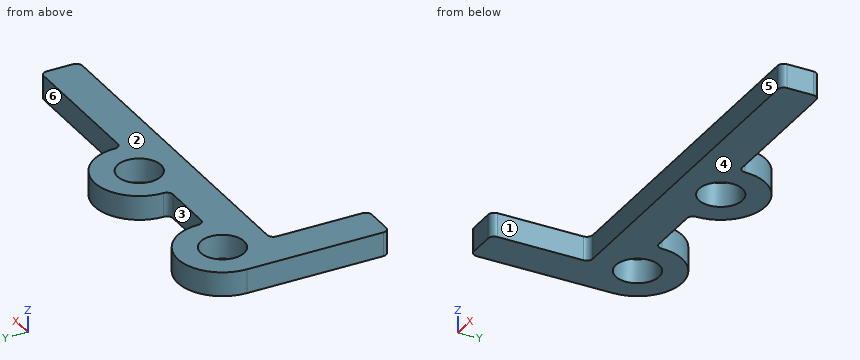
from build123d import *

# Parameters (mm, degrees)
SKETCH005_R = 1.8
PAD_DEPTH   = 2


with BuildPart() as part:
    # Sketch005 → Pad (new body)
    with BuildSketch(Plane.XY):
        with BuildLine():
            Line((121.287, -283.168), (121.287, -290.28))
            ThreePointArc((120.779, -290.788), (121.13821, -290.63921), (121.287, -290.28))
            Line((120.779, -290.788), (118.598, -290.788))
            ThreePointArc((118.09, -290.28), (118.23879, -290.63921), (118.598, -290.788))
            Line((118.09, -290.28), (118.09, -278.955))
            ThreePointArc((125.5, -278.955), (121.795, -275.25), (118.09, -278.955))
            ThreePointArc((125.5, -278.955), (125.64879, -279.31421), (126.008, -279.463))
            Line((126.008, -279.463), (130.282, -279.463))
            ThreePointArc((130.282, -279.463), (130.64121, -279.31421), (130.79, -278.955))
            ThreePointArc((138.2, -278.955), (134.495, -275.25), (130.79, -278.955))
            ThreePointArc((138.2, -278.955), (138.34879, -279.31421), (138.708, -279.463))
            Line((138.708, -279.463), (149.987, -279.463))
            ThreePointArc((150.495, -279.971), (150.34621, -279.61179), (149.987, -279.463))
            Line((150.495, -282.152), (150.495, -279.971))
            ThreePointArc((149.987, -282.66), (150.34621, -282.51121), (150.495, -282.152))
            Line((121.795, -282.66), (149.987, -282.66))
            ThreePointArc((121.795, -282.66), (121.43579, -282.80879), (121.287, -283.168))
        make_face()
        with Locations((121.795, -278.955)):
            Circle(SKETCH005_R, mode=Mode.SUBTRACT)
        with Locations((134.495, -278.955)):
            Circle(SKETCH005_R, mode=Mode.SUBTRACT)
    extrude(amount=PAD_DEPTH)


solid = part.part
Could you check a few things on this model? Use its own coordinates, in mm. Face numbers are marked on the shaded views. A direction names the side the tool comes from. Round coordinates to 2 decimals unless told otherwise and drop trailing zeros. Order: outer loops, then holes, each group sorted by start corner. A loop starts at its lowest first (then second) coordinate and runs counter-clockwise, first axis right, second up.
Q1. Thinking about a two-plate mould opening in X: for the marked faces 1, 2 and 3, which applies, released by +X, released by -X, zero draft, split by the parting line, or undercut?
Geometry says:
face 1: released by +X
face 2: zero draft
face 3: undercut
Q2. Which directions (+Z, -Z, +X, -X, +Y, -Y) give clear straight access to the entire face, cutting with the end or side of a thin tool? Please do the marked faces 4, 5 and 6.
Geometry says:
face 4: -Z, +X, -X, +Y, -Y
face 5: +Z, -Z, +X, -Y
face 6: +Z, -Z, +X, +Y
Q3. Imagine slicing it at B-B, the plane x = 147.5. List the corners of the cut face in (y, z) for me.
Geometry says:
outline: (-282.66, 0) - (-279.46, 0) - (-279.46, 2) - (-282.66, 2) - close
Q4. I'm going to push flat-ended pins straight in: P1, Ø0.6, axis at x = 129, z = 1.5, coming from the +Y side; P2, Ø0.6, axis at y = -287.5, z = 0.5, coming from the +X side. Where does each tip first touch, or does it pass through?
Geometry says:
P1: stops at y = -279.46
P2: stops at x = 121.29
Q5. Please list where these lines run through material, in increasing order: probe 1 along X at (y, z) = (-278, 0.3); probe 2 along Y at (x, z) = (147, 1.1); probe 3 along X at (y, z) = (-284, 0.6).
Geometry says:
probe 1: x = 118.22 to 120.27, 123.32 to 125.37, 130.92 to 132.97, 136.02 to 138.07
probe 2: y = -282.66 to -279.46
probe 3: x = 118.09 to 121.29
Q6. Imagine slicing it at A-A, the plane z = 1.2. List the corners of the cut face in (x, y) for me (3 decimals).
Geometry says:
outline: (118.09, -290.28) arc R0.508 ccw to (118.598, -290.788) - (120.779, -290.788) arc R0.508 ccw to (121.287, -290.28) - (121.287, -283.168) arc R0.508 cw to (121.795, -282.66) - (149.987, -282.66) arc R0.508 ccw to (150.495, -282.152) - (150.495, -279.971) arc R0.508 ccw to (149.987, -279.463) - (138.708, -279.463) arc R0.508 cw to (138.2, -278.955) arc R3.705 ccw to (130.79, -278.955) arc R0.508 cw to (130.282, -279.463) - (126.008, -279.463) arc R0.508 cw to (125.5, -278.955) arc R3.705 ccw to (118.09, -278.955) - close; hole circle Ø3.6 at (121.795, -278.955); hole circle Ø3.6 at (134.495, -278.955)
Q7. Imagine slicing it at C-C, the plane y = -284.25. List the corners of the cut face in (x, z) for me.
Geometry says:
outline: (118.09, 0) - (121.29, 0) - (121.29, 2) - (118.09, 2) - close
